```python
from build123d import *

# Parameters (mm, degrees)
PAD_DEPTH       = 0.1
PAD001_DEPTH    = 2.2
PAD002_DEPTH    = 1
PAD003_DEPTH    = 28
POCKET_DEPTH    = 8
SKETCH005_W     = 5
SKETCH005_H     = 3
POCKET001_DEPTH = 60
CHAMFER_SIZE    = 3.4
CHAMFER001_SIZE = 0.5


with BuildPart() as part:
    # Sketch → Pad (new body)
    with BuildSketch(Plane.XY):
        Polygon((0, 0), (60, 0), (72, -13), (59, -26), (0, -26), align=None)
    extrude(amount=PAD_DEPTH)

    # Sketch001 (on Face7 of Pad) → Pad001 (join)
    with BuildSketch(Plane.XY.offset(0.1)):
        Polygon((0, -1), (59.5, -1), (70.5, -13), (58.5, -25), (0.001879, -25), (0, -26), (59, -26), (72, -13), (60, 0), (0, 0), align=None)
    extrude(amount=PAD001_DEPTH)

    # Sketch002 (on Face3 of Pad001) → Pad002 (join)
    with BuildSketch(Plane.XY.offset(2.3)):
        Polygon((0, 0), (60, 0), (72, -13), (59, -26), (0, -26), align=None)
    extrude(amount=PAD002_DEPTH)

    # Sketch003 (on Face9 of Pad002) → Pad003 (join)
    with BuildSketch(Plane.XY.offset(3.3)):
        Polygon((2, -9), (68.307692, -9), (72, -13), (69, -16), (2, -16), align=None)
    extrude(amount=PAD003_DEPTH)

    # Sketch004 (on Face13 of Pad003) → Pocket (cut)
    with BuildSketch(Plane.XZ.offset(16)):
        Polygon((2, 31.3), (72, 6.3), (72, 31.3), align=None)
    extrude(amount=-POCKET_DEPTH, mode=Mode.SUBTRACT)

    # Sketch005 (on Face7 of Pocket) → Pocket001 (cut)
    with BuildSketch(Plane(origin=(0, 0, 0), x_dir=(0, -1, 0), z_dir=(-1, 0, 0))):
        with Locations((12.5, 3.8)):
            Rectangle(SKETCH005_W, SKETCH005_H)
    extrude(amount=-POCKET001_DEPTH, mode=Mode.SUBTRACT)

    # Chamfer
    chamfer_edges = [part.edges().sort_by_distance(p)[0] for p in [
        (35.153846, -9, 19.459341),
        (35.5, -16, 19.335714),
    ]]
    chamfer(chamfer_edges, length=CHAMFER_SIZE)

    # Chamfer001
    chamfer001_edges = [part.edges().sort_by_distance(p)[0] for p in [
        (35.5, -16, 3.3),
        (35.153846, -9, 3.3),
    ]]
    chamfer(chamfer001_edges, length=CHAMFER001_SIZE)


solid = part.part
```
The model under review builds one solid part; all positions refer to its coordinate system, in mm. A direction names the side the tool comes from. Give positions to 0.01 mm unless a question says otherwise; leave off trailing zeros. Loops run counter-clockwise (first coordinate to the right, second up) from the corner with the lowest first, then second, coordinate; pieces in that order, holes last. Notation, with made-up numbers: (51, -30) -> (66, -30) arc R17 cw to (66, -22) -> close; hole circle Ø8 at (64, 16.5). An arc over 180 degrees is marked (long way). Use CSV: the item, a comma, the result in double quotes.
1. To check wall thickness, follow probe 1 along Y at (x, z) = (21, 11); probe 2 along Z at (x, y) = (62.5, -22.25); probe 3 along Y at (x, z) = (64, 8). State the ranges of each line that lie inside material, in increasing order. Write a range as from..to.
Result:
probe 1,"y = -16..-9"
probe 2,"z = 0..3.3"
probe 3,"y = -13.69..-11.31"
2. Machinability: for faces 4 (the face through (27, -9, 13)), 5 (the face through (65, -7, 1)), 6 (the face through (2, -12, 17)), which of the approach directions +Z, -Z, +X, -X, +Y, -Y give a long, thin tool a straight path to every point of the face, cutting with its end or side? Answer none if there is none.
Result:
face 4,"+Z, +X, -X, +Y"
face 5,"-X"
face 6,"+Z, -X, +Y, -Y"
3. For P1, Ø6.5, axis at y = -11, z = 14, coming from the -X side; P2, Ø8, axis at x = 23.5, z = 25, coming from the +Y side; P3, Ø0.9, axis at x = 25.5, z = 4, coming from the +Y side, all flat-tipped, find the tip position at first contact; note any pin that passes through.
Result:
P1,"stops at x = 2"
P2,"stops at y = -9.7"
P3,"stops at y = -8.75"
4. Consider section C-C, the plane z = 17.5. Write out the cut boundary in (x, y).
Result:
outline,"(2, -16) -> (30.53, -16) -> (40.64, -12.6) -> (40.64, -12.4) -> (30.53, -9) -> (2, -9) -> close"
5. Consider section A-A, the plane x = 18. Write out the cut boundary in (y, z), then the cut area to 3 significant figures.
Result:
outline,"(-26, 0) -> (0, 0) -> (0, 3.3) -> (-8.5, 3.3) -> (-9, 3.8) -> (-9, 21.98) -> (-12.4, 25.59) -> (-12.6, 25.59) -> (-16, 21.98) -> (-16, 3.8) -> (-16.5, 3.3) -> (-26, 3.3) -> close; hole (-25, 0.1) -> (-1, 0.1) -> (-1, 2.3) -> (-10, 2.3) -> (-10, 5.3) -> (-15, 5.3) -> (-15, 2.3) -> (-25, 2.3) -> close"
area,"162 mm²"
6. Consider section B-B, the plane y = -22. Write out the cut boundary in (x, z).
Result:
outline,"(0, 0) -> (63, 0) -> (63, 3.3) -> (0, 3.3) -> (0, 2.3) -> (61.5, 2.3) -> (61.5, 0.1) -> (0, 0.1) -> close"
7. The part is to be moulded in two halves that separate along Y. For faces 1 (the face through (66, -19, 2)), 2 (the face through (35, -20, 3.3)), 3 (the face through (64.6, -18.9, 1.2)), say which applies: +Y half, -Y half, draft (parallel to the pull), parting line (faces both ways), or undercut.
Result:
face 1,"-Y half"
face 2,"draft"
face 3,"undercut"
8. Consider section D-D, the plane x = 36. Write out the cut boundary in (y, z), then the cut area to 3 significant figures.
Result:
outline,"(-26, 0) -> (0, 0) -> (0, 3.3) -> (-8.5, 3.3) -> (-9, 3.8) -> (-9, 15.55) -> (-12.4, 19.16) -> (-12.6, 19.16) -> (-16, 15.55) -> (-16, 3.8) -> (-16.5, 3.3) -> (-26, 3.3) -> close; hole (-25, 0.1) -> (-1, 0.1) -> (-1, 2.3) -> (-10, 2.3) -> (-10, 5.3) -> (-15, 5.3) -> (-15, 2.3) -> (-25, 2.3) -> close"
area,"117 mm²"
